from build123d import *

# Parameters (mm, degrees)
SKETCH1_R           = 75.9206
BOSS_EXTRUDE1_DEPTH = 12.7
SKETCH1_10_R        = 40.4114
CUT_EXTRUDE2_DEPTH  = 13.7
CUT_EXTRUDE5_DEPTH  = 6.35


with BuildPart() as part:
    # Sketch1 → Boss-Extrude1 (new body)
    with BuildSketch(Plane(origin=(0, 0, 0), x_dir=(1, 0, 0), z_dir=(0, 1, 0))):
        Circle(SKETCH1_R)
    extrude(amount=BOSS_EXTRUDE1_DEPTH)

    # Sketch1<10> → Cut-Extrude2 (cut, through all)
    with BuildSketch(Plane(origin=(0, 0, 0), x_dir=(1, 0, 0), z_dir=(0, 1, 0))):
        Circle(SKETCH1_10_R)
    extrude(amount=CUT_EXTRUDE2_DEPTH, mode=Mode.SUBTRACT)

    # Sketch3 → Cut-Extrude5 (cut)
    with BuildSketch(Plane(origin=(0, 12.7, 0), x_dir=(1, 0, 0), z_dir=(0, 1, 0))):
        Polygon((-28.180043708, 25.701493018), (-25.701493019, 28.180043708), (-60.52670499, 63.00525568), (-63.00525568, 60.52670499), align=None)
        Polygon((28.180043708, 25.701493019), (63.00525568, 60.52670499), (60.52670499, 63.00525568), (25.701493019, 28.180043708), align=None)
        Polygon((25.701493019, -28.180043708), (60.52670499, -63.00525568), (63.00525568, -60.52670499), (28.180043708, -25.701493018), align=None)
        Polygon((-28.180043708, -25.701493019), (-63.00525568, -60.52670499), (-60.52670499, -63.00525568), (-25.701493018, -28.180043708), align=None)
    extrude(amount=-CUT_EXTRUDE5_DEPTH, mode=Mode.SUBTRACT)


solid = part.part
Geometry: final body of the model. Coordinates: model frame, mm. A direction names the side the tool comes from. Round coordinates to 2 decimals unless told otherwise and drop trailing zeros. Loops run counter-clockwise (first coordinate to the right, second up) from the corner with the lowest first, then second, coordinate; pieces in that order, holes last.
Q1. Section C-C on z = 0. Return loops of the section in (x, y).
Q2. Access query for faces 1 (the flat face through (-40.046, 9.569, 42.524)), 2 (the flat face through (33, 0, 33)). Directions: +Z, -Z, +X, -X, +Y, -Y. A direction counts if a zero-diameter tool reaches every point of the face in a straight line with its end or side. Return the directions, or none.
Q3. Section B-B on x = 0. Return loops of the section in (y, z).
Q4. Pin query (flat end, axial travel): P1, Ø1.5, axis at x = 57, y = 6, coming from the -Z side; P2, Ø2, axis at y = 5.5, z = 26, coming from the -X side; P3, Ø2, axis at y = 3.5, z = -52.5, coming from the +X side. Return the tip coordinate at first contact, or that it passes through.
Q5. Section A-A on y = 8.5. Return loops of the section in (x, z).
Q6. Material intervals for L1, parallel to Z at x = 0, y = 5.5; L2, parallel to Z at x = -15, y = 5, sorted ascending.
Q7. Pull-direction query (X, two-part tool) for faces 3 (the flat face through (-39.69, 9.57, -42.17)), 4 (the cylindrical face through (-60.248, 6.261, 46.197)), 5 (the flat face through (-1, 12.7, 53)); classes: released by +X, released by -X, zero draft, split by the parting line, or undercut.
Evaluation:
1. outline: (-75.92, 0) - (-40.41, 0) - (-40.41, 12.7) - (-75.92, 12.7) - close; (40.41, 0) - (75.92, 0) - (75.92, 12.7) - (40.41, 12.7) - close
2. face 1: +Y
2. face 2: +Z, -Z, +X, -X, -Y
3. outline: (0, -75.92) - (12.7, -75.92) - (12.7, -40.41) - (0, -40.41) - close; (0, 40.41) - (12.7, 40.41) - (12.7, 75.92) - (0, 75.92) - close
4. P1: stops at z = -50.99
4. P2: stops at x = -71.69
4. P3: stops at x = 55.78
5. outline: (-54.91, -52.43) - (-29.79, -27.31) arc R40.41 cw to (-29.79, 27.31) - (-54.91, 52.43) arc R75.92 ccw to start; (-52.43, -54.91) arc R75.92 ccw to (52.43, -54.91) - (27.31, -29.79) arc R40.41 cw to (-27.31, -29.79) - close; (-52.43, 54.91) - (-27.31, 29.79) arc R40.41 cw to (27.31, 29.79) - (52.43, 54.91) arc R75.92 ccw to start; (29.79, -27.31) - (54.91, -52.43) arc R75.92 ccw to (54.91, 52.43) - (29.79, 27.31) arc R40.41 cw to start
6. L1: z = -75.92 to -40.41, 40.41 to 75.92
6. L2: z = -74.42 to -37.52, 37.52 to 74.42
7. face 3: undercut
7. face 4: split by the parting line
7. face 5: zero draft
